Can you work these out from the model? Positions are in its coordinate system, mm. A direction names the side the tool comes from. Give positions to 0.01 mm unless a question says otherwise; leave off trailing zeros. Loops run counter-clockwise (first coordinate to the right, second up) from the corner with the lowest first, then second, coordinate; pieces in that order, holes last. Notation, with made-up numbers: (55.25, 40.5) -> (102.25, 40.5) arc R25 cw to (102.25, 77.5) -> close; hole circle Ø4 at (-23.5, -22.75). An arc over 180 degrees is marked (long way). Use CSV: the item, a comma, the result in double quotes.
from build123d import *

# Parameters (mm, degrees)
SKETCH_R    = 3.45
PAD_DEPTH   = 5
SKETCH001_R = 2.65
HOLE_DEPTH  = 5.001


with BuildPart() as part:
    # Sketch → Pad (new body, symmetric)
    with BuildSketch(Plane.XY):
        with BuildLine():
            ThreePointArc((-14.7, -35), (0, -49.7), (14.7, -35))
            Line((14.7, -35), (14.7, -5))
            Line((25, -5), (14.7, -5))
            Line((25, 0), (25, -5))
            Line((-25, 0), (25, 0))
            Line((-25, 0), (-25, -5))
            Line((-25, -5), (-14.7, -5))
            Line((-14.7, -5), (-14.7, -35))
        make_face()
        with Locations((-4.879037, -30.120963)):
            Circle(SKETCH_R, mode=Mode.SUBTRACT)
        with Locations((4.879037, -30.120963)):
            Circle(SKETCH_R, mode=Mode.SUBTRACT)
        with Locations((4.879037, -39.879037)):
            Circle(SKETCH_R, mode=Mode.SUBTRACT)
        with Locations((-4.879037, -39.879037)):
            Circle(SKETCH_R, mode=Mode.SUBTRACT)
    extrude(amount=PAD_DEPTH, both=True)

    # Sketch001 → Hole (cut, through all)
    with BuildSketch(Plane.XZ.offset(5)):
        with Locations((-19.85, 0)):
            Circle(SKETCH001_R)
        with Locations((19.85, 0)):
            Circle(SKETCH001_R)
    extrude(amount=-HOLE_DEPTH, mode=Mode.SUBTRACT)


solid = part.part
(1) If I drill on L1, parallel to Z at x = -19.85, y = -1.3; L2, parallel to Y at x = 2.5, z = -4; L3, parallel to X at y = -28, z = -3.75, over which ranges is the centre line in solid material (lowest first)? Write a range as from..to.
Answer sheet:
L1,"z = -5..-2.65, 2.65..5"
L2,"y = -49.49..-42.38, -37.38..-32.62, -27.62..0"
L3,"x = -14.7..-7.6, -2.16..2.16, 7.6..14.7"
(2) If we section it at B-B, the plane z = -1.5: Write out the boundary of the cut face in (x, y), then the cut area to 3 significant figures.
Answer sheet:
outline,"(-25, -5) -> (-22.03, -5) -> (-22.03, 0) -> (-25, 0) -> close; (-17.67, -5) -> (-14.7, -5) -> (-14.7, -35) arc R14.7 ccw to (14.7, -35) -> (14.7, -5) -> (17.67, -5) -> (17.67, 0) -> (-17.67, 0) -> close; (22.03, -5) -> (25, -5) -> (25, 0) -> (22.03, 0) -> close; hole circle Ø6.9 at (-4.88, -39.88); hole circle Ø6.9 at (-4.88, -30.12); hole circle Ø6.9 at (4.88, -39.88); hole circle Ø6.9 at (4.88, -30.12)"
area,"1,280 mm2"
(3) We'd pull the mould along Y, two halves only. Please class faces 1 (the face through (4.43, -36.46, -0.07)), 2 (the face through (-17.6, -5, 2.3)), 3 (the face through (0, 0, 0)): released by +Y, released by -Y, zero draft, split by the parting line, or undercut.
Answer sheet:
face 1,"undercut"
face 2,"released by -Y"
face 3,"released by +Y"
(4) Which directions (+Z, -Z, +X, -X, +Y, -Y) give clear straight access to the entire face, cutting with the end or side of a thin tool? Please do faces 4 (the face through (0, -19, 5)), 5 (the face through (14.7, -20, 0)), 6 (the face through (-14.7, -20, 0)).
Answer sheet:
face 4,"+Z, +X, -X, +Y, -Y"
face 5,"+Z, -Z, +X, -Y"
face 6,"+Z, -Z, -X, -Y"
(5) If we section it at C-C, the plane y = -29: Write out the boundary of the cut face in (x, z), then the cut area to 3 significant figures.
Answer sheet:
outline,"(-14.7, -5) -> (-8.14, -5) -> (-8.14, 5) -> (-14.7, 5) -> close; (-1.62, -5) -> (1.62, -5) -> (1.62, 5) -> (-1.62, 5) -> close; (8.14, -5) -> (14.7, -5) -> (14.7, 5) -> (8.14, 5) -> close"
area,"163 mm2"
(6) If we section it at D-D, the plane z = 1.75: Write out the boundary of the cut face in (x, y).
Answer sheet:
outline,"(-25, -5) -> (-21.84, -5) -> (-21.84, 0) -> (-25, 0) -> close; (-17.86, -5) -> (-14.7, -5) -> (-14.7, -35) arc R14.7 ccw to (14.7, -35) -> (14.7, -5) -> (17.86, -5) -> (17.86, 0) -> (-17.86, 0) -> close; (21.84, -5) -> (25, -5) -> (25, 0) -> (21.84, 0) -> close; hole circle Ø6.9 at (-4.88, -39.88); hole circle Ø6.9 at (-4.88, -30.12); hole circle Ø6.9 at (4.88, -39.88); hole circle Ø6.9 at (4.88, -30.12)"
(7) If we section it at A-A, the plane x = -19.85: Write out the boundary of the cut face in (y, z).
Answer sheet:
outline,"(-5, -5) -> (0, -5) -> (0, -2.65) -> (-5, -2.65) -> close; (-5, 2.65) -> (0, 2.65) -> (0, 5) -> (-5, 5) -> close"
(8) Will these pins go through, and if not, where does the flat tip stop? pin 1 Ø3 at (x, z) = (22, 2.5) entering from -Y; pin 2 Ø2 at (y, z) = (-18.5, 1) entering from -X; pin 3 Ø2 at (y, z) = (-28, -3) entering from +X.
Answer sheet:
pin 1,"stops at y = -5"
pin 2,"stops at x = -14.7"
pin 3,"stops at x = 14.7"
